Read the model definition and answer for the solid it produces. Units are mm, in the model's axes. Face numbers are marked on the shaded views. Round coordinates to 2 decimals unless told otherwise and drop trailing zeros. Order: outer loops, then holes, each group sorted by start corner. A loop starts at its lowest first (then second) coordinate and runs counter-clockwise, first axis right, second up. Notation, with made-up numbers: (-4.75, -29) - (46.25, -29) arc R29 cw to (46.25, -9) - close; hole circle Ø9 at (20, 26.5). An arc over 180 degrees is marked (long way). Answer as a JSON object with one key per item and string values. Group by question number.
Q1. Given pin 1 Ø12 at (x, y) = (-100.5, 7.5) entering from -Z; pin 2 Ø8 at (x, y) = (-39, 17) entering from +Z, each flat-ended and moving along its own axis, determine where each tip first touches the part or whether it passes through.
Q2. The mould has two halves that part along X. Classify the marked faces 1, 2 and 3: pulls with the +X half, pulls with the -X half, needs draft (parallel to the pull), parting line crosses it, or undercut.
Q3. Consider line 1 (X direction, y = 27, z = 20); line 2 (Y direction, x = 39, z = 46); line 3 (Z direction, x = 321, y = 27.5). Determine where each line is inside the solid, lowest interval first.
Q4. A cutting plane is placed at A-A on y = 27. Determine the outline of the cut face in (x, z), and give its area (3 significant figures).
Q5. A cutting plane is placed at B-B on x = 25.5. Determine the outline of the cut face in (y, z), and give its area (3 significant figures).
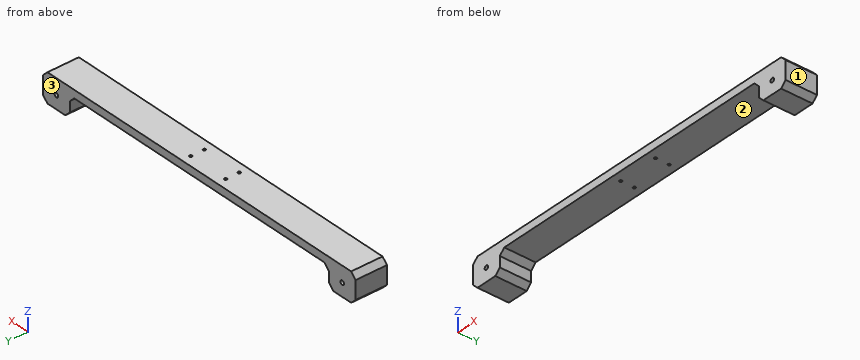
```python
from build123d import *

# Parameters (mm, degrees)
SKETCH2_R           = 4
BOSS_EXTRUDE2_DEPTH = 60
CHAMFER3_SIZE       = 10
SKETCH3_R           = 2.5
CUT_EXTRUDE1_DEPTH  = 360.339672177


with BuildPart() as part:
    # Sketch2 → Boss-Extrude2 (new body)
    with BuildSketch(Plane(origin=(0, 0, 0), x_dir=(1, 0, 0), z_dir=(0, 1, 0))):
        Polygon((-290, 5), (-350, 5), (-350, -50), (350, -50), (350, 5), (290, 5), (290, -35), (-290, -35), align=None)
        with Locations(Location((-320, -20, 0), (0, 0, 270))):
            Circle(SKETCH2_R, mode=Mode.SUBTRACT)
        with Locations(Location((320, -20, 0), (0, 0, 270))):
            Circle(SKETCH2_R, mode=Mode.SUBTRACT)
    extrude(amount=BOSS_EXTRUDE2_DEPTH)

    # Chamfer3
    chamfer3_edges = [part.edges().sort_by_distance(p)[0] for p in [
        (290, 30, -5),
        (350, 30, -5),
        (350, 30, 50),
        (-350, 30, 50),
        (-350, 30, -5),
        (-290, 30, -5),
        (-290, 30, 35),
        (290, 30, 35),
    ]]
    chamfer(chamfer3_edges, length=CHAMFER3_SIZE)

    # Sketch3 → Cut-Extrude1 (cut, through all)
    with BuildSketch(Plane.XY.offset(50)):
        with Locations((39, 43)):
            Circle(SKETCH3_R)
        with Locations(Location((39, 17, 0), (0, 0, 180))):
            Circle(SKETCH3_R)
        with Locations((-39, 17)):
            Circle(SKETCH3_R)
        with Locations(Location((-39, 43, 0), (0, 0, 180))):
            Circle(SKETCH3_R)
    extrude(amount=-CUT_EXTRUDE1_DEPTH, mode=Mode.SUBTRACT)


solid = part.part
```
Result set:
{
 "1": {"pin 1": "stops at z = 35", "pin 2": "stops at z = 50"},
 "2": {"face 1": "pulls with the +X half", "face 2": "undercut", "face 3": "needs draft"},
 "3": {"line 1": "x = -350 to -324, -316 to -290, 290 to 316, 324 to 350", "line 2": "y = 0 to 14.5, 19.5 to 40.5, 45.5 to 60", "line 3": "z = -5 to 16.13, 23.87 to 50"},
 "4": {"outline": "(-350, 5) - (-340, -5) - (-300, -5) - (-290, 5) - (-290, 25) - (-280, 35) - (280, 35) - (290, 25) - (290, 5) - (300, -5) - (340, -5) - (350, 5) - (350, 40) - (340, 50) - (-340, 50) - (-350, 40) - close; hole circle Ø8 at (-320, 20); hole circle Ø8 at (320, 20)", "area": "15,000 mm²"},
 "5": {"outline": "(0, 35) - (60, 35) - (60, 50) - (0, 50) - close", "area": "900 mm²"}
}
